Design review of the part built by this model. Coordinates are the model's own, in mm. A direction names the side the tool comes from. Coordinates: 2 decimals unless noted, no trailing zeros. Loops run counter-clockwise (first coordinate to the right, second up) from the corner with the lowest first, then second, coordinate; pieces in that order, holes last. Notation, with made-up numbers: M 77.25,0 L 135.25,0 A29 cw 135.25,31 Z; hole C 11.5,-33 d1. An arc over 180 degrees is marked long. Answer as a JSON object with one key per item and string values. Group by question number.
1. Machinability: for faces 4 (the flat face through (8, -3, -3.175)), 5 (the flat face through (-8.5, -5.2, -2.1)), 6 (the flat face through (8.4, -5.3, -2)), 7 (the flat face through (4.233, -3, -2)), 8 (the flat face through (0, -6.35, -3)), which of the approach directions +Z, -Z, +X, -X, +Y, -Y give a long, thin tool a straight path to every point of the face, cutting with its end or side? Answer none if there is none.
2. Insertion check: pin 1 (1.5 mm diameter, centred on x = 10, y = -3.5, fed in from -Z) (3 decimals); pin 2 (1.3 mm diameter, centred on y = -5.5, z = -4, fed in from -X); pin 3 (0.8 mm diameter, centred on y = -1, z = -3.5, fed in from +X). Each pin has a flat end and moves straight along its axis. Give the tip position at first contact, or say it passes through.
3. Draft analysis for pull direction Z (two halves, no side actions). For faces 1 (the flat face through (-4.233, -3, -2)), 2 (the flat face through (0, -1, -10.033)), 3 (the cylindrical face through (0.178, -3.344, 1.536)), state which applies: +Z half, -Z half, draft (parallel to the pull), parting line (faces both ways), or undercut.
4. To check wall thickness, follow probe 1 along Y at (x, z) = (-3.5, -4.5); probe 2 along Z at (x, y) = (2, -3) (3 decimals); probe 3 along X at (y, z) = (-4.5, -4.25). State the ranges of each line that lie inside material, in increasing order.
5. Consider section C-C (z = -7.25). State the section outline as (x, y) points, then the cut area to 3 significant figures.
6. Consider section D-D (z = 2). State the section outline as (x, y) points, then the cut area to 3 significant figures.
7. Consider section B-B (y = -3). State the section outline as (x, z) points (3 decimals), then the cut area to 3 significant figures.
8. Consider section A-A (x = 0). Count the separate pieces of the cut face and the enclosed holes in it, then the cut area to 3 significant figures.
from build123d import *

# Parameters (mm, degrees)
F1_DEPTH = 6.35
F0_W     = 8.4666666667
F0_H     = 6.858
F2_DEPTH = 6.35
F3_SIZE  = 2.2225
F4_R     = 1.27
F5_T     = 2.54
F7_D     = 3.175
F7_DEPTH = 25.4
F7_TIP   = 0.9538662327
F9_D     = 1.27
F9_DEPTH = 25.4
F9_TIP   = 0.3815464931


# Not quite as in the source:
# - a shell that OpenCascade refuses in one call is made with other operations: the cavity is built on its own and cut out


with BuildPart() as f1:
    # F0 (on Front) → F1 (new body)
    with BuildSketch(Plane.XZ):
        Polygon((12.7, -3.175), (12.7, 3.175), (-12.7, 3.175), (-12.7, -3.175), (-4.2333333333, -3.175), (4.2333333333, -3.175), align=None)
    extrude(amount=F1_DEPTH)

    # F0 (on Front) → F2 (join)
    with BuildSketch(Plane.XZ):
        with Locations((0, -6.604)):
            Rectangle(F0_W, F0_H)
    extrude(amount=F2_DEPTH)

    # F3
    f3_edges = [f1.edges().sort_by_distance(p)[0] for p in [
        (0, -6.35, 3.175),
        (8.466667, -6.35, -3.175),
        (-8.466667, -6.35, -3.175),
        (0, 0, 3.175),
        (8.466667, 0, -3.175),
        (-8.466667, 0, -3.175),
    ]]
    chamfer(f3_edges, length=F3_SIZE)

    # F4
    f4_edges = [f1.edges().sort_by_distance(p)[0] for p in [
        (-4.233333, -3.175, -10.033),
        (4.233333, -3.175, -10.033),
    ]]
    fillet(f4_edges, radius=F4_R)

    # F5: shell of thickness 2.54, made by hand


with BuildPart() as f5_core1:
    # F5_t2: copy of F1
    add(f1.part)

    # the walls: a layer under each face that stays
    f5_faces = [f5_core1.faces().sort_by_distance(p)[0] for p in [
        (0, 0, -4.54025),
        (8.4666666667, -1.11125, -2.06375),
        (12.7, -3.175, 0),
        (0, -1.11125, 2.06375),
        (-12.7, -3.175, 0),
        (-8.4666666667, -1.11125, -2.06375),
        (0, -6.35, -4.54025),
        (8.4666666667, -3.175, -3.175),
        (8.4666666667, -5.23875, -2.06375),
        (0, -5.23875, 2.06375),
        (0, -3.175, 3.175),
        (-8.4666666667, -3.175, -3.175),
        (-8.4666666667, -5.23875, -2.06375),
    ]]
    thicken(f5_faces, amount=-F5_T, mode=Mode.SUBTRACT)


with BuildPart() as f1_1:
    add(f1.part)

    # what is left inside the walls is the cavity
    f5_cavity = [f5_core1.part.solids().sort_by_distance(p)[0] for p in [
        (0, -2.5654, -6.721867),
    ]]
    add(f5_cavity, mode=Mode.SUBTRACT)

    # F7
    with Locations(Plane(origin=(-12.7, 0, 0), x_dir=(0, -1, 0), z_dir=(-1, 0, 0))):
        with Locations((3.1371232575, -0.0378767425)):
            Hole(F7_D / 2, depth=F7_DEPTH)
            with Locations((0, 0, -(F7_DEPTH + F7_TIP / 2))):  # 118° drill point
                Cone(0, F7_D / 2, F7_TIP, mode=Mode.SUBTRACT)

    # F9
    with Locations(Plane.XZ.offset(6.35)):
        with Locations((0, -7.5871711597)):
            Hole(F9_D / 2, depth=F9_DEPTH)
            with Locations((0, 0, -(F9_DEPTH + F9_TIP / 2))):  # 118° drill point
                Cone(0, F9_D / 2, F9_TIP, mode=Mode.SUBTRACT)


solid = f1_1.part
Findings below:
{
 "1": {"face 4": "-Z, +X, +Y, -Y", "face 5": "-Z, -X, -Y", "face 6": "-Z, +X, -Y", "face 7": "-Z", "face 8": "+Z, -Z, +X, -X, -Y"},
 "2": {"pin 1": "stops at z = -3.175", "pin 2": "stops at x = -4.23", "pin 3": "stops at x = 4.23"},
 "3": {"face 1": "draft", "face 2": "-Z half", "face 3": "undercut"},
 "4": {"probe 1": "y = -6.35 to -3.81, -2.54 to 0", "probe 2": "z = 1.544 to 3.175", "probe 3": "x = -4.23 to 4.23"},
 "5": {"outline": "M -4.23,-6.35 L -0.54,-6.35 L -0.54,-3.81 L -4.23,-3.81 Z; M -4.23,-2.54 L -0.54,-2.54 L -0.54,0 L -4.23,0 Z; M 0.54,-6.35 L 4.23,-6.35 L 4.23,-3.81 L 0.54,-3.81 Z; M 0.54,-2.54 L 4.23,-2.54 L 4.23,0 L 0.54,0 Z", "area": "37.5 mm^2"},
 "6": {"outline": "M -12.7,-5.3 L 12.7,-5.3 L 12.7,-1.05 L -12.7,-1.05 Z", "area": "108 mm^2"},
 "7": {"outline": "M -12.7,-3.175 L -4.233,-3.175 L -4.233,-1.619 L -12.7,-1.619 Z; M -12.7,1.544 L 12.7,1.544 L 12.7,3.175 L -12.7,3.175 Z; M 4.233,-3.175 L 12.7,-3.175 L 12.7,-1.619 L 4.233,-1.619 Z", "area": "67.8 mm^2"},
 "8": {"separate pieces": "3", "enclosed holes": "0", "area": "53.8 mm^2"}
}
